CAD build for the part. Positions are in the model's coordinates, mm. A direction names the side the tool comes from. Round coordinates to 2 decimals unless told otherwise and drop trailing zeros. Loops run counter-clockwise (first coordinate to the right, second up) from the corner with the lowest first, then second, coordinate; pieces in that order, holes last.
from build123d import *

# Parameters (mm, degrees)
SKETCH1_W           = 10.16
SKETCH1_H           = 3.175
BOSS_EXTRUDE1_DEPTH = 4.445
BOSS_EXTRUDE2_DEPTH = 1.905
SKETCH3_OUTSIDE_W   = 15.188
SKETCH3_OUTSIDE_H   = 13.918
SKETCH3_OUTSIDE_W_2 = 10.16
SKETCH3_OUTSIDE_H_2 = 8.89
SKETCH3_OUTSIDE_W_3 = 5.08
SKETCH3_OUTSIDE_H_3 = 5.08
CUT_EXTRUDE1_DEPTH  = 1.905


with BuildPart() as part:
    # Sketch1 → Boss-Extrude1 (new body, symmetric)
    with BuildSketch(Plane.XY):
        with Locations((0, -1.5875)):
            Rectangle(SKETCH1_W, SKETCH1_H)
    extrude(amount=BOSS_EXTRUDE1_DEPTH, both=True)

    # Sketch2 → Boss-Extrude2 (add, symmetric)
    with BuildSketch(Plane.XY):
        with BuildLine():
            Line((-1.905, 2.834704526), (-1.905, 3.681371192))
            Line((-1.905, 3.681371192), (-2.394734966, 3.681371192))
            ThreePointArc((-2.394734966, 3.681371192), (-2.382785125, 1.954968743), (-1.27, 0.635))
            Line((-1.27, 0.635), (-1.27, 0))
            Line((-1.27, 0), (1.27, 0))
            Line((1.27, 0), (1.27, 0.635))
            ThreePointArc((1.27, 0.635), (2.382785125, 1.954968743), (2.394734966, 3.681371192))
            Line((2.394734966, 3.681371192), (1.905, 3.681371192))
            Line((1.905, 3.681371192), (1.905, 2.834704526))
            ThreePointArc((1.905, 2.834704526), (0, 0.929704526), (-1.905, 2.834704526))
        make_face()
    extrude(amount=BOSS_EXTRUDE2_DEPTH, both=True)

    # Sketch3 outside → Cut-Extrude1 (cut)
    with BuildSketch(Plane.XZ.offset(3.175)):
        Rectangle(SKETCH3_OUTSIDE_W, SKETCH3_OUTSIDE_H)
        Rectangle(SKETCH3_OUTSIDE_W_2, SKETCH3_OUTSIDE_H_2, mode=Mode.SUBTRACT)
        Rectangle(SKETCH3_OUTSIDE_W_3, SKETCH3_OUTSIDE_H_3)
    extrude(amount=-CUT_EXTRUDE1_DEPTH, mode=Mode.SUBTRACT)


solid = part.part
Item 1: Cut at C-C (y = 2). List the corners of the cut face in (x, z) (3 decimals), plus the area to 3 significant figures.
Verdict:
outline: (-2.399, -1.905) - (-1.712, -1.905) - (-1.712, 1.905) - (-2.399, 1.905) - close; (1.712, -1.905) - (2.399, -1.905) - (2.399, 1.905) - (1.712, 1.905) - close
area: 5.23 mm2
Item 2: Cut at A-A (z = 0.75). List the corners of the cut face in (x, y) (3 decimals).
Verdict:
outline: (-5.08, -3.175) - (-2.54, -3.175) - (-2.54, -1.27) - (2.54, -1.27) - (2.54, -3.175) - (5.08, -3.175) - (5.08, 0) - (1.27, 0) - (1.27, 0.635) arc R2.54 ccw to (2.395, 3.681) - (1.905, 3.681) - (1.905, 2.835) arc R1.905 cw to (-1.905, 2.835) - (-1.905, 3.681) - (-2.395, 3.681) arc R2.54 ccw to (-1.27, 0.635) - (-1.27, 0) - (-5.08, 0) - close
Item 3: Cut at D-D (z = 4). List the corners of the cut face in (x, y) (3 decimals).
Verdict:
outline: (-5.08, -3.175) - (5.08, -3.175) - (5.08, 0) - (-5.08, 0) - close
Item 4: Wall check: L1, parallel to Z at x = 0.25, y = -1.75 (3 decimals); L2, parallel to X at y = -2.5, z = 0.5; L3, parallel to Y at x = -3, z = -1.5 (3 decimals). Give the ranges that are in metal, low to high.
Verdict:
L1: z = -4.445 to -2.54, 2.54 to 4.445
L2: x = -5.08 to -2.54, 2.54 to 5.08
L3: y = -3.175 to 0
Item 5: Mould opens along Z. For faces 4 (the flat face through (0.18, 0.76, 1.905)), 5 (the cylindrical face through (0.04, 0.93, 0.03)), 6 (the flat face through (0.18, 0.76, -1.905)), 7 (the flat face through (0, -2, -2.54)) say: released by +Z, released by -Z, zero draft, split by the parting line, or undercut.
Verdict:
face 4: released by +Z
face 5: zero draft
face 6: released by -Z
face 7: undercut
Item 6: Flat gauge pins, fed straight in: P1, Ø4, axis at x = -1, z = 1.5, coming from the -Y side (3 decimals); P2, Ø1.1, axis at x = -1, y = 2.5, coming from the +Z side; P3, Ø2.5, axis at x = 0.5, z = -0.5, coming from the -Y side; P4, Ø0.9, axis at y = 3.5, z = 1, coming from the +X side. Where does each tip first touch, or does it go through?
Verdict:
P1: stops at y = -3.175
P2: passes through
P3: stops at y = -1.27
P4: stops at x = 2.53
Item 7: Cut at B-B (x = 0). List the corners of the cut face in (y, z) (3 decimals), plus the area to 3 significant figures.
Verdict:
outline: (-3.175, -4.445) - (0, -4.445) - (0, -1.905) - (0.93, -1.905) - (0.93, 1.905) - (0, 1.905) - (0, 4.445) - (-3.175, 4.445) - (-3.175, 2.54) - (-1.27, 2.54) - (-1.27, -2.54) - (-3.175, -2.54) - close
area: 22.1 mm2
Item 8: 3-axis set-ups, long thin cutter, end or side, ignore diameter. For faces 1 (the flat face through (0, -2, 2.54)), 2 (the cylindrical face through (2.374, 1.932, 0.027)), 3 (the flat face through (-1.905, 3, 0)): which of +Z, -Z, +X, -X, +Y, -Y reach the whole face in a straight line?
Verdict:
face 1: -Y
face 2: +Z, -Z, +X
face 3: +Z, -Z, +Y
